```python
from build123d import *

# Parameters (mm, degrees)
BOSS_EXTRUDE1_DEPTH = 100
SKETCH2_R           = 3
BOSS_EXTRUDE2_DEPTH = 10
SKETCH3_R           = 3
CUT_EXTRUDE1_DEPTH  = 12


with BuildPart() as part:
    # Sketch1 → Boss-Extrude1 (new body)
    with BuildSketch(Plane(origin=(0, 0, 0), x_dir=(1, 0, 0), z_dir=(0, 1, 0))):
        Polygon((0, -5.773502692), (5, -2.886751346), (5, 2.886751346), (0, 5.773502692), (-5, 2.886751346), (-5, -2.886751346), align=None)
    extrude(amount=BOSS_EXTRUDE1_DEPTH)

    # Sketch2 → Boss-Extrude2 (add)
    with BuildSketch(Plane(origin=(0, 100, 0), x_dir=(1, 0, 0), z_dir=(0, 1, 0))):
        Circle(SKETCH2_R)
    extrude(amount=BOSS_EXTRUDE2_DEPTH)

    # Sketch3 → Cut-Extrude1 (cut)
    with BuildSketch(Plane.XZ):
        Circle(SKETCH3_R)
    extrude(amount=-CUT_EXTRUDE1_DEPTH, mode=Mode.SUBTRACT)


solid = part.part
```
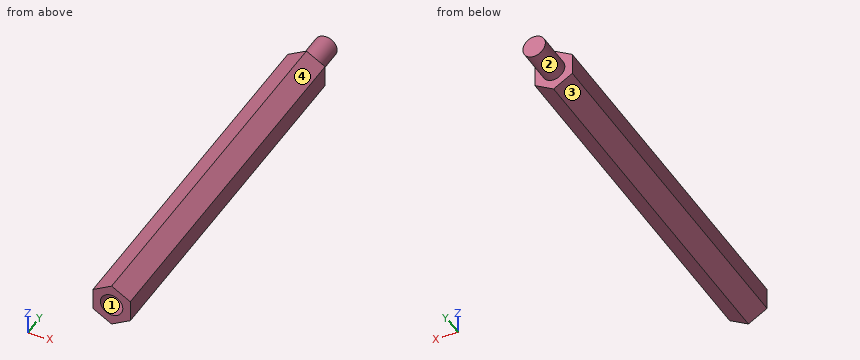
Input: part model. Units: mm. Frame: model coordinates. Face numbers are marked on the shaded views. Give positions to 0.01 mm unless a question says otherwise; leave off trailing zeros. Order: outer loops, then holes, each group sorted by start corner. A loop starts at its lowest first (then second) coordinate and runs counter-clockwise, first axis right, second up. Notation, with made-up numbers: M -6.75,55 L 28.25,55 A21 cw 28.25,67 Z; hole C 79,-38.5 d3. An arc over 180 degrees is marked long. Return JSON: item names as keys, results as strings.
Item 1: Cut plane B-B (y = 26). Return loops of the section in (x, z).
Solutions:
{"outline": "M -5,-2.89 L 0,-5.77 L 5,-2.89 L 5,2.89 L 0,5.77 L -5,2.89 Z"}
Item 2: Cut plane A-A (z = 0). Return loops of the section in (x, y), then the cut area to 3 significant figures.
Solutions:
{"outline": "M -5,0 L -3,0 L -3,12 L 3,12 L 3,0 L 5,0 L 5,100 L 3,100 L 3,110 L -3,110 L -3,100 L -5,100 Z", "area": "988 mm^2"}
Item 3: First-contact query: P1, Ø6, axis at x = -0.5, z = 1.5, coming from the -Y side; P2, Ø1.8, axis at x = 0, z = 1, coming from the -Y side. Flat tips, straight axial feed; report the tip coordinate or a pass-through.
Solutions:
{"P1": "y = 0", "P2": "y = 12"}
Item 4: Pull-direction query (X, two-part tool) for the marked faces 1, 2, 3 and 4; classes: +X half, -X half, draft (parallel to the pull), parting line (faces both ways), or undercut.
Solutions:
{"face 1": "undercut", "face 2": "parting line", "face 3": "-X half", "face 4": "+X half"}
Item 5: Ray query, probe 1 along Z at (x, y) = (0, 9.25); probe 2 along Y at (x, z) = (-1.25, -1.5); probe 3 along Y at (x, z) = (-4, 2.5). Return the intervals inside material, ascending.
Solutions:
{"probe 1": "-5.77 to -3, 3 to 5.77", "probe 2": "12 to 110", "probe 3": "0 to 100"}
